Check sheet for the modelled part. Datum: model origin and axes. Units: mm. A direction names the side the tool comes from. Round coordinates to 2 decimals unless told otherwise and drop trailing zeros. Order: outer loops, then holes, each group sorted by start corner. A loop starts at its lowest first (then second) coordinate and runs counter-clockwise, first axis right, second up.
Q1. Cross-section at D-D on y = 9. Record the cut outline in (x, z), then the cut area to 3 significant figures.
Q2. Cross-section at C-C on y = 45. Record the cut outline in (x, z), then the cut area to 3 significant figures.
Q3. Set-up check for faces 1 (the cylindrical face through (0.878, 2.242, 3.954)), 2 (the flat face through (0, 0, 0)): record each of +Z, -Z, +X, -X, +Y, -Y from which the full face is reachable in a straight line by a thin tool's end or side.
Q4. Depth check by flat-ended pin: P1, Ø1.5, axis at x = -1.5, z = 5.5, coming from the -Y side; P2, Ø1, axis at y = 17, z = -2, coming from the -X side; P3, Ø1, axis at x = 1.5, y = 38.5, coming from the +Z side; P4, Ø3, axis at x = 2.5, z = 1, coming from the -Y side. Enter the tip coordinate at first touch or a pass-through.
Q5. Scan lines: probe 1 along X at (y, z) = (47.5, -1.25); probe 2 along Y at (x, z) = (-2, -0.25); probe 3 along X at (y, z) = (10.5, 3.5). Record each from-to range of solid material in increasing order.
from build123d import *

# Parameters (mm, degrees)
CHAMFER1_SIZE2 = 1
CHAMFER1_SIZE  = 0.577350269


with BuildPart() as part:
    # Sketch1 → Revolve1 (revolve)
    with BuildSketch(Plane.XY, mode=Mode.PRIVATE) as revolve1_sk:
        with BuildLine():
            Line((0, 0), (4.05, 0))
            Line((4.05, 0), (4.05, 5))
            Line((4.05, 5), (5.05, 5))
            Line((5.05, 5), (5.05, 7))
            ThreePointArc((5.05, 7), (5.529083978, 26.391142635), (7.88435805, 45.644677848))
            ThreePointArc((7.88435805, 45.644677848), (6.117294223, 52.155454528), (0, 55))
            Line((0, 55), (0, 0))
        make_face()
    revolve(revolve1_sk.sketch.rotate(Axis((0, 55, 0), (0, -1, 0)), 180), axis=Axis((0, 55, 0), (0, -1, 0)))

    # Chamfer1
    chamfer1_edges = [part.edges().sort_by_distance(p)[0] for p in [
        (4.05, 5, 0),
    ]]
    chamfer1_side = [part.faces().sort_by_distance(p)[0] for p in [
        (4.05, 4.988452995, 0),
    ]]
    chamfer(chamfer1_edges, length=CHAMFER1_SIZE - 0.0001, length2=CHAMFER1_SIZE2 - 0.0001, reference=chamfer1_side[0])  # a hair under: the kernel refuses the full size


solid = part.part
Results found:
1. outline: circle Ø10.02 at (0, 0)
1. area: 78.9 mm2
2. outline: circle Ø15.55 at (0, 0)
2. area: 190 mm2
3. face 1: -Y
3. face 2: +Z, -Z, +X, -X, -Y
4. P1: stops at y = 4.94
4. P2: stops at x = -4.84
4. P3: stops at z = 6.74
4. P4: stops at y = 0
5. probe 1: x = -7.89 to 7.89
5. probe 2: y = 0 to 54.74
5. probe 3: x = -3.57 to 3.57
